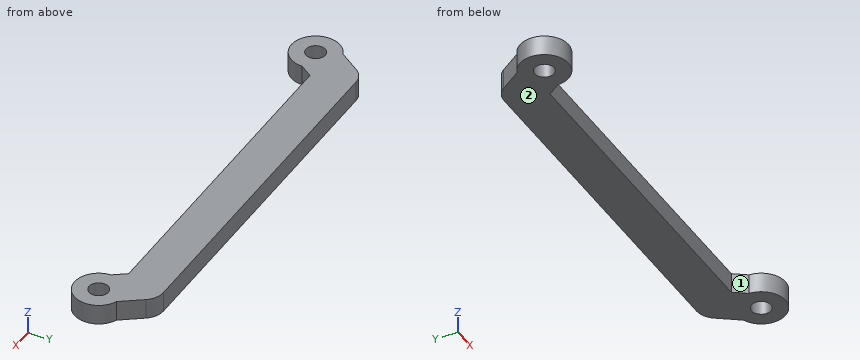
```python
from build123d import *

# Parameters (mm, degrees)
SKETCH1_R           = 1.2
BOSS_EXTRUDE1_DEPTH = 1.25
SKETCH2_R           = 3
SKETCH2_R_2         = 1.2
BOSS_EXTRUDE2_DEPTH = 2.5


with BuildPart() as part:
    # Sketch1 → Boss-Extrude1 (new body, symmetric)
    with BuildSketch(Plane.XY):
        with BuildLine():
            Line((-20.897752221, 1.5), (20.897752221, 1.5))
            Line((20.897752221, 1.5), (22.952119889, -1.433941091))
            ThreePointArc((22.952119889, -1.433941091), (26.433941091, -2.047880111), (27.047880111, 1.433941091))
            Line((27.047880111, 1.433941091), (24.247049958, 5.433941091))
            ThreePointArc((24.247049958, 5.433941091), (23.35354138, 6.217527083), (22.199169847, 6.5))
            Line((22.199169847, 6.5), (-22.199169847, 6.5))
            ThreePointArc((-22.199169847, 6.5), (-23.35354138, 6.217527083), (-24.247049958, 5.433941091))
            Line((-24.247049958, 5.433941091), (-27.047880111, 1.433941091))
            ThreePointArc((-27.047880111, 1.433941091), (-26.433941091, -2.047880111), (-22.952119889, -1.433941091))
            Line((-22.952119889, -1.433941091), (-20.897752221, 1.5))
        make_face()
        with Locations((-25, 0)):
            Circle(SKETCH1_R, mode=Mode.SUBTRACT)
        with Locations((25, 0)):
            Circle(SKETCH1_R, mode=Mode.SUBTRACT)
    extrude(amount=BOSS_EXTRUDE1_DEPTH, both=True)

    # Sketch2 → Boss-Extrude2 (add)
    with BuildSketch(Plane(origin=(0, 0, -1.25), x_dir=(-1, 0, 0), z_dir=(0, 0, -1))):
        with Locations((25, 0)):
            Circle(SKETCH2_R)
        with Locations((25, 0)):
            Circle(SKETCH2_R_2, mode=Mode.SUBTRACT)
        with Locations((-25, 0)):
            Circle(SKETCH2_R)
        with Locations((-25, 0)):
            Circle(SKETCH2_R_2, mode=Mode.SUBTRACT)
    extrude(amount=-BOSS_EXTRUDE2_DEPTH)


solid = part.part
```
Geometry: final body of the model. Coordinates: model frame, mm. Face numbers are marked on the shaded views. A direction names the side the tool comes from. Coordinates: 2 decimals unless noted, no trailing zeros. Order: outer loops, then holes, each group sorted by start corner. A loop starts at its lowest first (then second) coordinate and runs counter-clockwise, first axis right, second up. Notation, with made-up numbers: (21, 12.5) - (67, 12.5) arc R25 ccw to (67, 27.5) - close; hole circle Ø8 at (0.25, 77.5). An arc over 180 degrees is marked (long way). Return JSON: item names as keys, results as strings. Group by question number.
1. Cut plane D-D (x = 14). Output: boundary loops of the cut face in (y, z).
2. Cut plane C-C (x = 25). Output: boundary loops of the cut face in (y, z), plus the area to 3 significant figures.
3. Cut plane A-A (z = 0.6). Output: boundary loops of the cut face in (x, y).
4. Material intervals for line 1 along X through (y, z) = (0, 0.75); line 2 along X through (y, z) = (-1, 0.4); line 3 along Y through (x, z) = (-10, 0.8), sorted ascending. Write a range as [from, to].
5. Pin query (flat end, axial travel): pin 1 (0.8 mm diameter, centred on x = -6.5, z = 0.5, fed in from -Y). Return the tip coordinate at first contact, or that it passes through.
6. Set-up query: the marked faces 1 and 2. Return all of +Z, -Z, +X, -X, +Y, -Y with unobstructed straight access to the full face (end or side cutting, diameter ignored); none if empty.
7. Cut plane B-B (y = -1.75). Output: boundary loops of the cut face in (x, z), plus the area to 3 significant figures.
Resolved:
{
 "1": {"outline": "(1.5, -1.25) - (6.5, -1.25) - (6.5, 1.25) - (1.5, 1.25) - close"},
 "2": {"outline": "(-3, -1.25) - (-1.2, -1.25) - (-1.2, 1.25) - (-3, 1.25) - close; (1.2, -1.25) - (4.36, -1.25) - (4.36, 1.25) - (1.2, 1.25) - close", "area": "12.4 mm²"},
 "3": {"outline": "(-26.1, 2.79) arc R3 ccw (long way) to (-22, -0.08) - (-20.9, 1.5) - (20.9, 1.5) - (22, -0.08) arc R3 ccw (long way) to (26.1, 2.79) - (24.25, 5.43) arc R2.5 ccw to (22.2, 6.5) - (-22.2, 6.5) arc R2.5 ccw to (-24.25, 5.43) - close; hole circle Ø2.4 at (-25, 0); hole circle Ø2.4 at (25, 0)"},
 "4": {"line 1": "x = [-28, -26.2], [-23.8, -21.95], [21.95, 23.8], [26.2, 28]", "line 2": "x = [-27.83, -25.66], [-24.34, -22.17], [22.17, 24.34], [25.66, 27.83]", "line 3": "y = [1.5, 6.5]"},
 "5": {"pin 1": "stops at y = 1.5"},
 "6": {"face 1": "+Z, -Z, -Y", "face 2": "-Z, +X, -X, +Y, -Y"},
 "7": {"outline": "(-27.44, -1.25) - (-22.56, -1.25) - (-22.56, 1.25) - (-27.44, 1.25) - close; (22.56, -1.25) - (27.44, -1.25) - (27.44, 1.25) - (22.56, 1.25) - close", "area": "24.4 mm²"}
}
